from build123d import *

# Parameters (mm, degrees)
SZKIC1_W                    = 125
SZKIC1_H                    = 55
SZKIC1_R                    = 7.5
DODANIE_WYCI_GNI_CIE1_DEPTH = 10
SZKIC2_W                    = 20
SZKIC2_H                    = 55
DODANIE_WYCI_GNI_CIE2_DEPTH = 45
WYTNIJ_WYCI_GNI_CIE1_DEPTH  = 45


with BuildPart() as part:
    # Szkic1 → Dodanie-wyciągnięcie1 (new body)
    with BuildSketch(Plane.XY):
        Rectangle(SZKIC1_W, SZKIC1_H)
        with Locations((-37.5, 0)):
            Circle(SZKIC1_R, mode=Mode.SUBTRACT)
        with Locations((37.5, 0)):
            Circle(SZKIC1_R, mode=Mode.SUBTRACT)
    extrude(amount=DODANIE_WYCI_GNI_CIE1_DEPTH)

    # Szkic2 → Dodanie-wyciągnięcie2 (add)
    with BuildSketch(Plane.XY.offset(10)):
        Rectangle(SZKIC2_W, SZKIC2_H)
    extrude(amount=DODANIE_WYCI_GNI_CIE2_DEPTH)

    # Szkic3 → Wytnij-wyciągnięcie1 (cut)
    with BuildSketch(Plane(origin=(10, 0, 0), x_dir=(0, 0, -1), z_dir=(1, 0, 0))):
        Polygon((-55, -12.5), (-10, 27.5), (-55, 27.5), align=None)
    extrude(amount=-WYTNIJ_WYCI_GNI_CIE1_DEPTH, mode=Mode.SUBTRACT)


solid = part.part
For this review, take the finished solid that the model builds, in its own axes (mm). A direction names the side the tool comes from. Coordinates: 2 decimals unless noted, no trailing zeros. Order: outer loops, then holes, each group sorted by start corner. A loop starts at its lowest first (then second) coordinate and runs counter-clockwise, first axis right, second up. Notation, with made-up numbers: (-9.75, 34.5) - (6.25, 34.5) arc R3 ccw to (6.25, 39.5) - close; hole circle Ø1 at (21.25, 59). An arc over 180 degrees is marked (long way). Use one line per item in the form item = value.
Q1. Consider section D-D (x = -4). Give the boundary of the cut face in (y, z), then the cut area to 4 significant figures.
Checked values:
outline = (-27.5, 0) - (27.5, 0) - (27.5, 10) - (-12.5, 55) - (-27.5, 55) - close
area = 2,125 mm2
Q2. For P1, Ø17, axis at x = -37.5, y = 0, coming from the +Z side; P2, Ø10, axis at y = -11, z = 27.5, coming from the +X side, all flat-tipped, find the tip position at first contact; note any pin that passes through.
Checked values:
P1 = 10
P2 = 10
Q3. For faces 5 (the flat face through (-42.5, 6.5, 10)), 6 (the flat face through (62.5, 0, 5)), 7 (the flat face through (10, -6, 27)), list the 3-axis set-ups (+Z, -Z, +X, -X, +Y, -Y) from which the entire face can be reached by the end or side of a thin tool; tool diameter is ignored.
Checked values:
face_5 = +Z, -X, +Y, -Y
face_6 = +Z, -Z, +X, +Y, -Y
face_7 = +Z, +X, +Y, -Y
Q4. Consider section A-A (x = -37.5). Give the boundary of the cut face in (y, z), then the cut area to 3 significant figures.
Checked values:
outline = (-27.5, 0) - (-7.5, 0) - (-7.5, 10) - (-27.5, 10) - close; (7.5, 0) - (27.5, 0) - (27.5, 10) - (7.5, 10) - close
area = 400 mm2
Q5. Consider section C-C (y = -18). Give the boundary of the cut face in (x, z), then the cut area to 3 significant figures.
Checked values:
outline = (-62.5, 0) - (62.5, 0) - (62.5, 10) - (10, 10) - (10, 55) - (-10, 55) - (-10, 10) - (-62.5, 10) - close
area = 2,150 mm2
Q6. Consider section B-B (y = -2.5). Give the boundary of the cut face in (x, z).
Checked values:
outline = (-62.5, 0) - (-44.57, 0) - (-44.57, 10) - (-62.5, 10) - close; (-30.43, 0) - (30.43, 0) - (30.43, 10) - (10, 10) - (10, 43.75) - (-10, 43.75) - (-10, 10) - (-30.43, 10) - close; (44.57, 0) - (62.5, 0) - (62.5, 10) - (44.57, 10) - close
Q7. For probe 1 along Y at (x, z) = (37.5, 4.75); probe 2 along Z at (x, y) = (-56, 2); probe 3 along Z at (x, y) = (6.5, 10.5) (3 decimals), list the stretches that pass through material, from the lowest coordinate up. Write a range as from..to.
Checked values:
probe_1 = -27.5..-7.5, 7.5..27.5
probe_2 = 0..10
probe_3 = 0..29.125
Q8. Draft analysis for pull direction Y (two halves, no side actions). For faces 1 (the cylindrical face through (30, 0, 5)), 2 (the flat face through (-1, 27.5, 5)), 3 (the flat face through (0, -20, 55)), 4 (the flat face through (0, -27.5, 19)), state which applies: +Y half, -Y half, draft (parallel to the pull), parting line (faces both ways), or undercut.
Checked values:
face_1 = undercut
face_2 = +Y half
face_3 = draft
face_4 = -Y half
